Could you check a few things on this drawing? It's one solid part, dimensions in mm from its lowest x, y, z. A direction names the side the tool comes from. Coordinates: 2 decimals unless noted, no trailing zeros. Write each loop counter-clockwise with the first axis right and the second up, starting at its lowest first coordinate (ties: lowest second). Pieces come first, ordered by that corner, then holes.
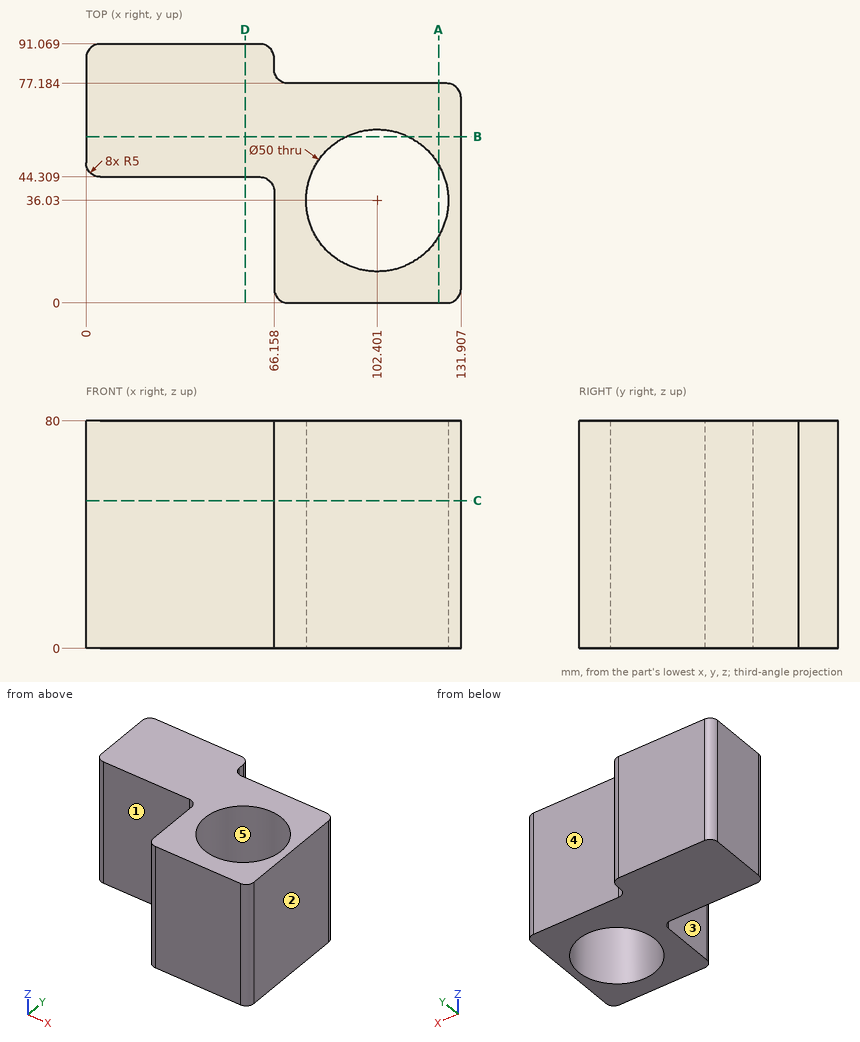
1) Will these pins go through, and if not, where does the flat tip stop? pin 1 (10.5 mm diameter, centred on y = 22.5, z = 23.5, fed in from -X); pin 2 (16.5 mm diameter, centred on x = 87, z = 51, fed in from +Y); pin 3 (1.9 mm diameter, centred on y = 83.5, z = 20.5, fed in from +X).
Values follow:
pin 1: stops at x = 66.16
pin 2: stops at y = 77.18
pin 3: stops at x = 66.16
2) We'd pull the mould along Y, two halves only. Please class the marked faces 3, 4 and 5: pulls with the +Y half, pulls with the -Y half, needs draft (parallel to the pull), parting line crosses it, or undercut.
Values follow:
face 3: needs draft
face 4: pulls with the +Y half
face 5: undercut
3) Imagine slicing it at D-D on x = 56. Please give me the cut outline in (y, z), then the cut area to 3 significant figures.
Values follow:
outline: (44.31, 0) - (91.07, 0) - (91.07, 80) - (44.31, 80) - close
area: 3,740 mm2
4) Imagine slicing it at A-A on x = 124. Please give me the cut outline in (y, z).
Values follow:
outline: (0, 0) - (23.44, 0) - (23.44, 80) - (0, 80) - close; (48.62, 0) - (77.18, 0) - (77.18, 80) - (48.62, 80) - close
5) Imagine slicing it at C-C on z = 52. Please give me the cut outline in (x, y), then the cut area to 3 significant figures.
Values follow:
outline: (0, 49.31) arc R5 ccw to (5, 44.31) - (61.16, 44.31) arc R5 cw to (66.16, 39.31) - (66.16, 5) arc R5 ccw to (71.16, 0) - (126.91, 0) arc R5 ccw to (131.91, 5) - (131.91, 72.18) arc R5 ccw to (126.91, 77.18) - (71.16, 77.18) arc R5 cw to (66.16, 82.18) - (66.16, 86.07) arc R5 ccw to (61.16, 91.07) - (5, 91.07) arc R5 ccw to (0, 86.07) - close; hole circle Ø50 at (102.4, 36.03)
area: 6,180 mm2
6) On a 3-axis mill with a long thin cutter (end or side, diameter ignored), from which of +Z, -Z, +X, -X, +Y, -Y can I reach the whole of each face in a straight line? I mean the marked faces 1 and 2. Say none if no direction works.
Values follow:
face 1: +Z, -Z, -X, -Y
face 2: +Z, -Z, +X, +Y, -Y
7) Imagine slicing it at B-B on y = 58.5. Please give me the cut outline in (x, z).
Values follow:
outline: (0, 0) - (91.44, 0) - (91.44, 80) - (0, 80) - close; (113.36, 0) - (131.91, 0) - (131.91, 80) - (113.36, 80) - close
8) I need wall thicknesses on probe 1 along X at (y, z) = (35.5, 14) (1 decimal); probe 2 along Y at (x, z) = (101.5, 28.5); probe 3 along Y at (x, z) = (7, 42). Which ranges of each line are inside material? Lowest first, please.
Values follow:
probe 1: x = 66.2 to 77.4, 127.4 to 131.9
probe 2: y = 0 to 11.05, 61.01 to 77.18
probe 3: y = 44.31 to 91.07
